The listing builds one solid part. Answer for the finished solid, in the listing's coordinates (mm). Round coordinates to 2 decimals unless told otherwise and drop trailing zeros. Write each loop counter-clockwise with the first axis right and the second up, starting at its lowest first coordinate (ties: lowest second). Pieces come first, ordered by that corner, then holes. Notation, with made-up numbers: (11, 89) - (49, 89) arc R18 ccw to (49, 109) - close; hole circle Ø9 at (25, 31). An arc over 180 degrees is marked (long way). Answer in a Markdown table with one row per item.
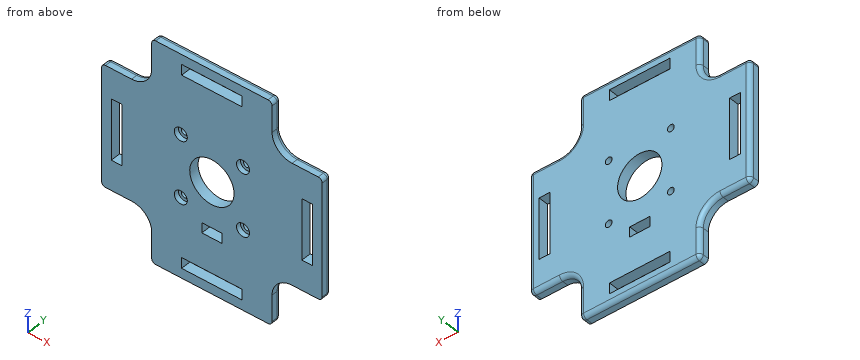
from build123d import *

# Parameters (mm, degrees)
BOSS_EXTRUDE1_DEPTH                                  = 5
CUT_EXTRUDE1_REACH                                   = 79.942
SKETCH2_R                                            = 11.05
SKETCH2_W                                            = 5.3
SKETCH2_H                                            = 30.2
CIRPATTERN1_COUNT                                    = 4
CBORE_FOR_M3_HEX_SOCKET_THIN_HEAD_CAP_SC_D           = 3.4
CBORE_FOR_M3_HEX_SOCKET_THIN_HEAD_CAP_SC_CBORE_D     = 6.5
CBORE_FOR_M3_HEX_SOCKET_THIN_HEAD_CAP_SC_CBORE_DEPTH = 2.4
FILLET1_R                                            = 10
FILLET2_R                                            = 2
FILLET3_R                                            = 2
CUT_EXTRUDE2_REACH                                   = 79.942
SKETCH6_W                                            = 10
SKETCH6_H                                            = 5


with BuildPart() as part:
    # Sketch1 → Boss-Extrude1 (new body)
    with BuildSketch(Plane(origin=(0, 0, 0), x_dir=(1, 0, 0), z_dir=(0, 1, 0))):
        Polygon((-30, 55), (30, 55), (30, 30), (55, 30), (55, -30), (30, -30), (30, -55), (-30, -55), (-30, -30), (-55, -30), (-55, 30), (-30, 30), align=None)
    extrude(amount=BOSS_EXTRUDE1_DEPTH)

    # Sketch2 → Cut-Extrude1 (cut, up to next)
    with BuildSketch(Plane(origin=(0, 5, 0), x_dir=(1, 0, 0), z_dir=(0, 1, 0)), mode=Mode.PRIVATE) as cut_extrude1_sk1:
        with Locations(Location((0, 0, 0), (0, 0, 270))):
            Circle(SKETCH2_R)
    cut_extrude1_tool1 = extrude(cut_extrude1_sk1.sketch, amount=-CUT_EXTRUDE1_REACH, mode=Mode.PRIVATE) & part.part
    # Sketch2 → Cut-Extrude1 (cut, up to next)
    with BuildSketch(Plane(origin=(0, 5, 0), x_dir=(1, 0, 0), z_dir=(0, 1, 0)), mode=Mode.PRIVATE) as cut_extrude1_sk2:
        with Locations((-47.5, 0)):
            Rectangle(SKETCH2_W, SKETCH2_H)
    cut_extrude1_tool2 = extrude(cut_extrude1_sk2.sketch, amount=-CUT_EXTRUDE1_REACH, mode=Mode.PRIVATE) & part.part
    cut_extrude1_1 = cut_extrude1_tool1.solids().sort_by_distance((0, 5, 0))[0]
    add(cut_extrude1_1, mode=Mode.SUBTRACT)
    cut_extrude1_2 = cut_extrude1_tool2.solids().sort_by_distance((-47.5, 5, 0))[0]
    add(cut_extrude1_2, mode=Mode.SUBTRACT)
    cut_extrude1 = cut_extrude1_1 + cut_extrude1_2  # Cut-Extrude1 as one shape, for the pattern or mirror that repeats it

    # CirPattern1: Cut-Extrude1 ×4 about axis
    cirpattern1_axis = Axis((0, 0, 0), (0, 1, 0))
    for i in range(1, CIRPATTERN1_COUNT):
        add(cut_extrude1.rotate(cirpattern1_axis, i * 360 / CIRPATTERN1_COUNT), mode=Mode.SUBTRACT)

    # CBORE for M3 Hex Socket Thin Head Cap Screw1 (through all)
    with Locations(Plane(origin=(-15.5, 0, 15.5), x_dir=(0, 0, -1), z_dir=(0, -1, 0))):
        with Locations((0, 0), (31, 0), (31, 31), (0, 31)):
            CounterBoreHole(CBORE_FOR_M3_HEX_SOCKET_THIN_HEAD_CAP_SC_D / 2, CBORE_FOR_M3_HEX_SOCKET_THIN_HEAD_CAP_SC_CBORE_D / 2, CBORE_FOR_M3_HEX_SOCKET_THIN_HEAD_CAP_SC_CBORE_DEPTH)

    # Fillet1
    fillet1_edges = [part.edges().sort_by_distance(p)[0] for p in [
        (30, 2.5, -30),
        (30, 2.5, 30),
        (-30, 2.5, 30),
        (-30, 2.5, -30),
    ]]
    fillet(fillet1_edges, radius=FILLET1_R)

    # Fillet2
    fillet2_edges = [part.edges().sort_by_distance(p)[0] for p in [
        (-30, 2.5, -55),
        (30, 2.5, -55),
        (55, 2.5, -30),
        (55, 2.5, 30),
        (30, 2.5, 55),
        (-30, 2.5, 55),
        (-55, 2.5, 30),
        (-55, 2.5, -30),
    ]]
    fillet(fillet2_edges, radius=FILLET2_R)

    # Fillet3
    fillet3_edges = [part.edges().sort_by_distance(p)[0] for p in [
        (-46.5, 5, -30),
        (30, 5, -46.5),
        (46.5, 5, 30),
        (-30, 5, 46.5),
        (-32.928932188, 5, -32.928932188),
        (32.928932188, 5, -32.928932188),
        (32.928932188, 5, 32.928932188),
        (-32.928932188, 5, 32.928932188),
        (-55, 5, 0),
        (-30, 5, -46.5),
        (-46.5, 5, 30),
        (0, 5, 55),
        (30, 5, 46.5),
        (55, 5, 0),
        (46.5, 5, -30),
        (0, 5, -55),
        (-29.414213562, 5, -54.414213562),
        (54.414213562, 5, -29.414213562),
        (29.414213562, 5, -54.414213562),
        (29.414213562, 5, 54.414213562),
        (54.414213562, 5, 29.414213562),
        (-54.414213562, 5, 29.414213562),
        (-29.414213562, 5, 54.414213562),
        (-54.414213562, 5, -29.414213562),
    ]]
    fillet(fillet3_edges, radius=FILLET3_R)

    # Sketch6 → Cut-Extrude2 (cut, up to next)
    with BuildSketch(Plane(origin=(0, 5, 0), x_dir=(1, 0, 0), z_dir=(0, 1, 0)), mode=Mode.PRIVATE) as cut_extrude2_sk1:
        with Locations((0, 25)):
            Rectangle(SKETCH6_W, SKETCH6_H)
    cut_extrude2_tool1 = extrude(cut_extrude2_sk1.sketch, amount=-CUT_EXTRUDE2_REACH, mode=Mode.PRIVATE) & part.part
    add(cut_extrude2_tool1.solids().sort_by_distance((0, 5, -25))[0], mode=Mode.SUBTRACT)


solid = part.part
(1) Section D-D (y = 0.9) is taken. State how many separate pieces and enclosed holes the cut face has, and give its area (3 significant figures).
Checked values:
| item | result |
|---|---|
| separate pieces | 1 |
| enclosed holes | 10 |
| area | 8,470 mm2 |
(2) Section A-A (x = 0) is taken. Give the vertices of the cut face in (y, z).
Checked values:
| item | result |
|---|---|
| outline | (0, -55) - (3, -55) arc R2 ccw to (5, -53) - (5, -50.15) - (0, -50.15) - close; (0, -44.85) - (5, -44.85) - (5, -27.5) - (0, -27.5) - close; (0, -22.5) - (5, -22.5) - (5, -11.05) - (0, -11.05) - close; (0, 11.05) - (5, 11.05) - (5, 44.85) - (0, 44.85) - close; (0, 50.15) - (5, 50.15) - (5, 53) arc R2 ccw to (3, 55) - (0, 55) - close |
(3) Section C-C (z = 0) is taken. Give the vertices of the cut face in (x, y).
Checked values:
| item | result |
|---|---|
| outline | (-55, 0) - (-50.15, 0) - (-50.15, 5) - (-53, 5) arc R2 ccw to (-55, 3) - close; (-44.85, 0) - (-11.05, 0) - (-11.05, 5) - (-44.85, 5) - close; (11.05, 0) - (44.85, 0) - (44.85, 5) - (11.05, 5) - close; (50.15, 0) - (55, 0) - (55, 3) arc R2 ccw to (53, 5) - (50.15, 5) - close |
(4) Flat-ended cylindrical pins translate along their axes: pin 1 (1.5 mm diameter, centred on y = 3.5, z = -48.5, fed in from +X); pin 2 (2.5 mm diameter, centred on y = 2, z = 46.5, fed in from -X); pin 3 (0.9 mm diameter, centred on x = 48, y = 2, fed in from +Z). Find the tip coordinate at first contact, or state that the pin passes through.
Checked values:
| item | result |
|---|---|
| pin 1 | stops at x = 30 |
| pin 2 | stops at x = -30 |
| pin 3 | stops at z = 30 |
(5) Find the intervals of material crossed by line 1 (X direction, y = 2.65, z = 0); line 2 (X direction, y = 0.2, z = -25); line 3 (X direction, y = 3.75, z = 1), in increasing order.
Checked values:
| item | result |
|---|---|
| line 1 | x = -55 to -50.15, -44.85 to -11.05, 11.05 to 44.85, 50.15 to 55 |
| line 2 | x = -55 to -5, 5 to 55 |
| line 3 | x = -54.85 to -50.15, -44.85 to -11, 11 to 44.85, 50.15 to 54.85 |
(6) Section B-B (z = -24.5) is taken. Give the vertices of the cut face in (x, y), and give its area (3 significant figures).
Checked values:
| item | result |
|---|---|
| outline | (-55, 0) - (-5, 0) - (-5, 5) - (-53, 5) arc R2 ccw to (-55, 3) - close; (5, 0) - (55, 0) - (55, 3) arc R2 ccw to (53, 5) - (5, 5) - close |
| area | 498 mm2 |
